Here's how the part is built. I have some questions about the finished solid (model axes, mm). Face numbers are marked on the shaded views. Round coordinates to 2 decimals unless told otherwise and drop trailing zeros. Order: outer loops, then holes, each group sorted by start corner. A loop starts at its lowest first (then second) coordinate and runs counter-clockwise, first axis right, second up. Notation, with made-up numbers: (53, 30.5) -> (67, 30.5) arc R29 ccw to (67, 54.5) -> close; hole circle Ø3 at (44.25, -31). An arc over 180 degrees is marked (long way). One line per item, written item: value.
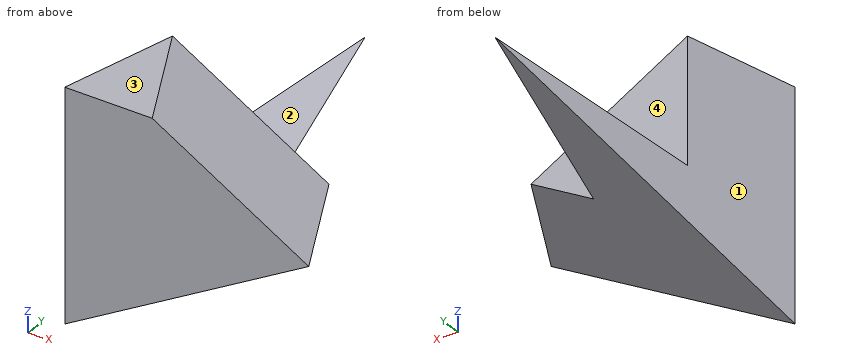
Autodesk Inventor part; units mm, degrees
ref_plane "YZ Plane" through (0, 0, 0) normal (1, 0, 0) x (0, 1, 0)
ref_plane "XZ Plane" through (0, 0, 0) normal (0, 1, 0) x (-1, 0, 0)
ref_plane "XY Plane" through (0, 0, 0) normal (0, 0, 1) x (1, 0, 0)
sketch "Эскиз1" plane through (0, 0, 0) normal (0, 1, 0) x (-1, 0, 0)
  line L0 (-24.9696, 12.6351) -> (42.5304, 51.6062)
  line L1 (42.5304, 51.6062) -> (42.5304, -26.3361)
  line L2 (42.5304, -26.3361) -> (-24.9696, 12.6351)
  point P0 (0, 0)
  point P1 (20.0304, 12.6351)
ref_plane "РабПлоскость2" through (0, 90, 0) normal (0, 1, 0) x (-1, 0, 0)
ref_plane "РабПлоскость1" through (0, 0, 0) normal (0, 1, 0) x (-1, 0, 0)
sketch "Эскиз3" plane through (0, 90, 0) normal (0, 1, 0) x (-1, 0, 0)
  point P0 (0, 0)
  point P1 (20.0304, 12.635)
loft "Лофт1" add profiles "Эскиз1" section 2 point at (-20.0304, 90, 12.635)
sketch "Эскиз4" plane through (0, 0, 0) normal (1, 0, 0) x (0, 1, 0)
  line L0 (0, 51.6062) -> (90, 12.635)
  line L1 (32.265, 37.6351) -> (32.265, 12.6351)
  line L2 (0, 12.6351) -> (90, 12.635)
  line L3 (32.265, 12.6351) -> (32.265, 2.6351)
  line L4 (0, -26.3361) -> (90, 12.635)
  line L5 (32.265, 2.6351) -> (90, 12.635)
  point P0 (0, 0)
  dimension "d6" = 25
  dimension "d7" = 10
extrude "Выдавливание1" cut sketch "Эскиз4" along normal mid plane 1000
sketch "Эскиз5" plane through (0, 0, 0) normal (1, 0, 0) x (0, 1, 0)
  line L0 (0, 51.6062) -> (32.265, 37.6351)
  line L1 (32.265, 37.6351) -> (0, 37.6351)
  line L2 (0, 51.6062) -> (0, -26.3361)
  point P0 (0, 0)
extrude "Выдавливание2" cut sketch "Эскиз5" along normal mid plane 100
Q1. I want a section at D-D on z = -15.5. Write out the boundary of the cut face in (x, y), then the cut area to 3 significant figures.
Answers:
outline: (-42.53, 0) -> (-23.76, 0) -> (-36.27, 25.02) -> close
area: 235 mm2
Q2. I want a section at B-B on x = -13. Write out the boundary of the cut face in (y, z) (3 decimals), then the cut area to 3 significant figures.
Answers:
outline: (0, -9.287) -> (54.848, 6.547) -> (32.265, 2.635) -> (32.265, 25.243) -> (0, 34.557) -> close
area: 1,140 mm2
Q3. For P1, Ø4, axis at x = -22, y = 45, coming from the +Z side; P2, Ø3, axis at x = -21.5, y = 42.5, coming from the +Z side; P3, Ø6, axis at x = 15, y = 10.5, coming from the +Z side; P4, Ø2, axis at x = -10.5, y = 48.5, coming from the -Z side, each with a flat end and sliding along its axis, tell me the tip position at first contact or that it passes through.
Answers:
P1: z = 5.19
P2: z = 4.67
P3: z = 17.3
P4: through
Q4. If we mould it in two halves opening along Y, with no side actions, what happens to the marked faces 1, 2, 3 and 4? For each: pulls with the +Y half, pulls with the -Y half, needs draft (parallel to the pull), parting line crosses it, or undercut.
Answers:
face 1: pulls with the +Y half
face 2: undercut
face 3: needs draft
face 4: undercut
Q5. I need wall thicknesses on line 1 along Y through (x, z) = (-24, 24) (3 decimals); line 2 along Z through (x, y) = (-13.5, 45); line 3 along X through (y, z) = (23, 18.5). Which ranges of each line are inside material? Lowest first, please.
Answers:
line 1: 0 to 32.265
line 2: 3.41 to 4.84
line 3: -36.78 to 3.31
Q6. I want a section at C-C on y = 29.5. Write out the boundary of the cut face in (x, z), then the cut area to 3 significant figures.
Answers:
outline: (-35.16, -13.56) -> (10.22, 12.64) -> (-33.08, 37.64) -> (-35.16, 37.64) -> close
area: 1,190 mm2
Q7. I want a section at A-A on z = 11. Write out the boundary of the cut face in (x, y) (3 decimals).
Answers:
outline: (-42.53, 0) -> (22.138, 0) -> (6.005, 32.265) -> (-34.464, 32.265) -> close; (-22.39, 80.56) -> (-18.142, 80.56) -> (-20.974, 86.224) -> close
